The listing builds one solid part. Answer for the finished solid, in the listing's coordinates (mm). Face numbers are marked on the shaded views. A direction names the side the tool comes from. Coordinates: 2 decimals unless noted, no trailing zeros. Order: outer loops, then holes, each group sorted by start corner. A loop starts at its lowest first (then second) coordinate and runs counter-clockwise, first axis right, second up. Notation, with made-up numbers: (31.5, -10) -> (45.5, -10) arc R22 cw to (45.5, -3) -> close; hole circle Ø7 at (-15.75, -3). An arc over 180 degrees is marked (long way). Put each result on its own line as item: value. Start each with the question number.
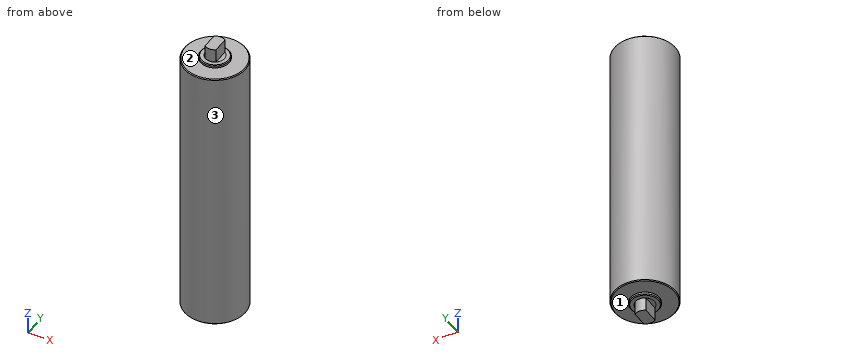
```python
from build123d import *

# Parameters (mm, degrees)
SKETCH1_R                = 55.753
EXTRUDE1_DEPTH           = 250.063
SKETCH2_R                = 26
EXTRUDE2_DEPTH           = 5.08
SKETCH3_R                = 17.5
EXTRUDE3_DEPTH           = 25.019
SKETCH4_W                = 7.467
SKETCH4_H                = 28.676743958
CUT_EXTRUDE1_DEPTH       = 24.892
CHAMFER1_SIZE            = 1.524
CHAMFER1_OF_MIRROR1_SIZE = 1.524


with BuildPart() as part:
    # Sketch1 → Extrude1 (new body)
    with BuildSketch(Plane.XY):
        Circle(SKETCH1_R)
    extrude1 = extrude(amount=EXTRUDE1_DEPTH)

    # Sketch2 → Extrude2 (add)
    with BuildSketch(Plane.XY.offset(250.063)):
        Circle(SKETCH2_R)
    extrude2 = extrude(amount=EXTRUDE2_DEPTH)

    # Sketch3 → Extrude3 (add)
    with BuildSketch(Plane.XY.offset(255.143)):
        Circle(SKETCH3_R)
    extrude3 = extrude(amount=EXTRUDE3_DEPTH)

    # Sketch4 → Cut-Extrude1 (cut)
    with BuildSketch(Plane.XY.offset(280.162)):
        with Locations((13.7665, 0)):
            Rectangle(SKETCH4_W, SKETCH4_H)
        with Locations((-13.7665, 0)):
            Rectangle(SKETCH4_W, SKETCH4_H)
    cut_extrude1 = extrude(amount=-CUT_EXTRUDE1_DEPTH, mode=Mode.SUBTRACT)

    # Chamfer1
    chamfer1_edges = [part.edges().sort_by_distance(p)[0] for p in [
        (-55.753, 0, 250.063),
        (-26, 0, 255.143),
    ]]
    chamfer(chamfer1_edges, length=CHAMFER1_SIZE)

    # Mirror1: Extrude1, Extrude2, Extrude3, Cut-Extrude1 across plane
    add(extrude1.mirror(Plane.XY))
    add(extrude2.mirror(Plane.XY))
    add(extrude3.mirror(Plane.XY))
    add(cut_extrude1.mirror(Plane.XY), mode=Mode.SUBTRACT)

    # Chamfer1 of Mirror1
    chamfer1_of_mirror1_edges = [part.edges().sort_by_distance(p)[0] for p in [
        (-55.753, 0, -250.063),
        (-26, 0, -255.143),
    ]]
    chamfer(chamfer1_of_mirror1_edges, length=CHAMFER1_OF_MIRROR1_SIZE)


solid = part.part
```
(1) Each of these flat-tipped pins is pushed along its axis until it touches: P1, Ø12.5, axis at y = 3, z = -263, coming from the +X side; P2, Ø12, axis at x = -42.5, y = -38, coming from the +Z side; P3, Ø20, axis at y = -4, z = 271, coming from the -X side; P4, Ø8, axis at x = 14, y = 0.5, coming from the -Z side. Where does it stop, or does it pass through?
(2) The part is cut by section B-B on z = -212.5. Determine the outline of the cut face in (x, y), plus the area to 3 significant figures.
(3) Find the intervals of material crossed by L1, parallel to X at y = -3, z = 101.5; L2, parallel to Z at x = -37, y = 6.5; L3, parallel to Y at x = 32.5, z = -80, in increasing order.
(4) A tool of negligible diameter and unlimited length cuts with its end or side. For the marked faces 1, 2 and 3, from which of +Z, -Z, +X, -X, +Y, -Y can it reach the whole face along a straight path? Write none if from no direction.
(5) The part is cut by section A-A on x = 0. Determine the outline of the cut face in (y, z).
Worked out:
1. P1: x = 10.03
1. P2: z = 250.06
1. P3: x = -10.03
1. P4: z = -280.16
2. outline: circle Ø111.51 at (0, 0)
2. area: 9,770 mm2
3. L1: -55.67 to 55.67
3. L2: -250.06 to 250.06
3. L3: -45.3 to 45.3
4. face 1: -Z
4. face 2: +Z
4. face 3: +Z, -Z
5. outline: (-55.75, -248.54) -> (-54.23, -250.06) -> (-26, -250.06) -> (-26, -253.62) -> (-24.48, -255.14) -> (-17.5, -255.14) -> (-17.5, -280.16) -> (17.5, -280.16) -> (17.5, -255.14) -> (24.48, -255.14) -> (26, -253.62) -> (26, -250.06) -> (54.23, -250.06) -> (55.75, -248.54) -> (55.75, 248.54) -> (54.23, 250.06) -> (26, 250.06) -> (26, 253.62) -> (24.48, 255.14) -> (17.5, 255.14) -> (17.5, 280.16) -> (-17.5, 280.16) -> (-17.5, 255.14) -> (-24.48, 255.14) -> (-26, 253.62) -> (-26, 250.06) -> (-54.23, 250.06) -> (-55.75, 248.54) -> close
